Here's how the part is built. I have some questions about the finished solid (model axes, mm). Give positions to 0.01 mm unless a question says otherwise; leave off trailing zeros. Loops run counter-clockwise (first coordinate to the right, second up) from the corner with the lowest first, then second, coordinate; pieces in that order, holes last. Notation, with made-up numbers: M 56,81.5 L 88,81.5 A21 cw 88,85.5 Z; hole C -15,59.25 d9. An arc over 180 degrees is marked long. Answer as CSV lines item,"result". Start each with the question number.
Item 1: If I drill on line 1 along X through (y, z) = (3.25, 95); line 2 along Z through (x, y) = (-0.25, 7); line 3 along Y through (x, z) = (4.75, 94), over which ranges is the centre line in solid material (lowest first)? Write a range as from..to.
Item 2: I want a section at A-A on z = 95. List the corners of the cut face in (x, y) for me.
Item 3: I want a section at B-B on x = 0. List the corners of the cut face in (y, z) for me.
Item 4: Will these pins go through, and if not, where does the flat tip stop? P1, Ø3, axis at x = -4, z = 70, coming from the +Y side; P2, Ø1.5, axis at x = -2, y = 12, coming from the -Z side.
Item 5: I want a section at D-D on y = 11.25. List the corners of the cut face in (x, z) for me, plus the area to 3 significant figures.
Item 6: I want a section at C-C on z = 5. List the corners of the cut face in (x, y) for me, plus the area to 3 significant figures.
Item 7: If we mould it in two halves opening along Z, with no side actions, what happens to faces 1 (the cylindrical face through (1.2, 9.9, 6.6)), 2 (the cylindrical face through (0.601, 0.07, 96.908)), 3 (the flat face through (5, 0, 49))? For each: released by +Z, released by -Z, zero draft, split by the parting line, or undercut.
from build123d import *

# Parameters (mm, degrees)
SKETCH2_W           = 10
SKETCH2_H           = 10
BOSS_EXTRUDE1_DEPTH = 100
CUT_EXTRUDE1_REACH  = 102.623
SKETCH3_R           = 2
SKETCH4_R           = 2
BOSS_EXTRUDE2_DEPTH = 10


with BuildPart() as part:
    # Sketch2 → Boss-Extrude1 (new body)
    with BuildSketch(Plane.XY):
        Rectangle(SKETCH2_W, SKETCH2_H)
    extrude(amount=BOSS_EXTRUDE1_DEPTH)

    # Sketch3 → Cut-Extrude1 (cut, up to next)
    with BuildSketch(Plane(origin=(0, 5, 0), x_dir=(1, 0, 0), z_dir=(0, 1, 0)), mode=Mode.PRIVATE) as cut_extrude1_sk1:
        with Locations(Location((0, -95, 0), (0, 0, 270))):
            Circle(SKETCH3_R)
    cut_extrude1_tool1 = extrude(cut_extrude1_sk1.sketch, amount=-CUT_EXTRUDE1_REACH, mode=Mode.PRIVATE) & part.part
    add(cut_extrude1_tool1.solids().sort_by_distance((0, 5, 95))[0], mode=Mode.SUBTRACT)

    # Sketch4 → Boss-Extrude2 (add)
    with BuildSketch(Plane(origin=(0, 5, 0), x_dir=(1, 0, 0), z_dir=(0, 1, 0))):
        with Locations(Location((0, -5, 0), (0, 0, 90))):
            Circle(SKETCH4_R)
    extrude(amount=BOSS_EXTRUDE2_DEPTH)


solid = part.part
Result:
1,line 1,"-5..-2, 2..5"
1,line 2,"3.02..6.98"
1,line 3,"-5..5"
2,outline,"M -5,-5 L -2,-5 L -2,5 L -5,5 Z; M 2,-5 L 5,-5 L 5,5 L 2,5 Z"
3,outline,"M -5,0 L 5,0 L 5,3 L 15,3 L 15,7 L 5,7 L 5,93 L -5,93 Z; M -5,97 L 5,97 L 5,100 L -5,100 Z"
4,P1,"y = 5"
4,P2,"z = 3.44"
5,outline,"C 0,5 d4"
5,area,"12.6 mm^2"
6,outline,"M -5,-5 L 5,-5 L 5,5 L 2,5 L 2,15 L -2,15 L -2,5 L -5,5 Z"
6,area,"140 mm^2"
7,face 1,"split by the parting line"
7,face 2,"undercut"
7,face 3,"zero draft"
